Build history of the part. All positions in model axes, mm. A direction names the side the tool comes from. Give positions to 0.01 mm unless a question says otherwise; leave off trailing zeros. Write each loop counter-clockwise with the first axis right and the second up, starting at its lowest first coordinate (ties: lowest second). Pieces come first, ordered by that corner, then holes. Notation, with made-up numbers: (27.25, 57.25) -> (82.25, 57.25) arc R23 cw to (82.25, 88.25) -> close; hole circle Ø4 at (41.5, -14). An arc over 180 degrees is marked (long way). Write item = value, one per line. Start each with the question number.
Q1. Tool access for faces 4 (the face through (-41.214, 41.905, 1.729)), 5 (the face through (135, -24, 11)), 6 (the face through (43.25, 42, 0)), 7 (the face through (155, -10, -10)): list every direction of +Z, -Z, +X, -X, +Y, -Y with a clear straight run to the whole face (end or side of a thin tool).
Q2. Saw through at B-B, the plane y = 21. List the corners of the cut face in (x, z).
Q3. Mould opens along X. For faces 1 (the face through (125.17, -29.38, 0.28)), 2 (the face through (37, 85, -6)), 3 (the face through (135, -24, -11)) say: pulls with the +X half, pulls with the -X half, needs draft (parallel to the pull), parting line crosses it, or undercut.
Q4. Saw through at D-D, the plane y = 53. List the corners of the cut face in (x, z).
Q5. Drop flat-ended pins along their axis: P1, Ø8, axis at x = 31.5, z = 3.5, coming from the -Y side; P2, Ø8, axis at x = 81, z = -21, coming from the +Y side; P3, Ø6.5, axis at x = 40.5, y = 33, coming from the +Z side; P4, Ø8, axis at y = 53, z = 12, coming from the -X side. Give the stop position or say it passes through.
Q6. Saw through at A-A, the plane z = 0. List the corners of the cut face in (x, y), then the cut area to 3 significant figures.
Q7. Wall check: line 1 (Z direction, x = 165, y = 3); line 2 (X direction, y = -20, z = 3); line 3 (X direction, y = -22, z = 10.5). Give the ranges that are in metal, low to high.
Q8. Saw through at C-C, the plane x = 0. List the corners of the cut face in (y, z).
from build123d import *

# Parameters (mm, degrees)
BOSS_EXTRUDE1_DEPTH     = 85
BOSS_EXTRUDE2_START     = -30
SKETCH2_3_R             = 12.5
BOSS_EXTRUDE2_DEPTH     = 56.666666667
EXTRUDE_THIN1_DEPTH     = 115
SKETCH5_W               = 50
SKETCH5_H               = 20
BOSS_EXTRUDE3_DEPTH     = 230
CUT_EXTRUDE2_DEPTH      = 311.201547385
CUT_EXTRUDE2_DEPTH_BACK = 311.201547385
SKETCH5_3_R             = 5
CUT_EXTRUDE1_START      = -30
CUT_EXTRUDE1_OUTLINE_R  = 8.5
CUT_EXTRUDE1_DEPTH      = 115
RIB1_START              = -2.5
RIB1_DEPTH              = 5
FILLET1_R               = 10


# Read off the part's stored shape, not the designer's step: Cut-Extrude1, Rib1
with BuildPart() as part:
    # Sketch2 → Boss-Extrude1 (new body)
    with BuildSketch(Plane(origin=(0, 0, 0), x_dir=(1, 0, 0), z_dir=(0, 1, 0))):
        with BuildLine():
            Line((40.811303581, 6), (46.25, 6))
            Line((46.25, 6), (46.25, -6))
            Line((46.25, -6), (40.811303581, -6))
            ThreePointArc((40.811303581, -6), (-41.25, 0), (40.811303581, 6))
        make_face()
    extrude(amount=BOSS_EXTRUDE1_DEPTH)



with BuildPart() as body_2:
    # Sketch2<3> → Boss-Extrude2 (new body)
    with BuildSketch(Plane(origin=(0, 0, 0), x_dir=(1, 0, 0), z_dir=(0, 1, 0)).offset(BOSS_EXTRUDE2_START)):
        with Locations(Location((165, 0, 0), (0, 0, 270))):
            Circle(SKETCH2_3_R)
    extrude(amount=BOSS_EXTRUDE2_DEPTH)


with BuildPart() as part_1:
    add(part.part)

    add(body_2.part)  # Extrude-Thin1 merges body 2
    # Sketch3 → Extrude-Thin1 (add, symmetric)
    with BuildSketch(Plane.XY):
        Polygon((-41.25, 0), (89.247392222, 0), (125, -30), (177.5, -30), (177.5, -24), (127.183821406, -24), (91.431213628, 6), (-41.25, 6), align=None)
    extrude(amount=EXTRUDE_THIN1_DEPTH, both=True)

    # Sketch5 → Boss-Extrude3 (add)
    with BuildSketch(Plane.XY.offset(115)):
        with Locations((165, -20)):
            Rectangle(SKETCH5_W, SKETCH5_H)
    extrude(amount=-BOSS_EXTRUDE3_DEPTH)

    # Sketch5<3> → Cut-Extrude2 (cut, two sides: drawn at the far end of the back side and taken through both)
    with BuildSketch(Plane.XY.offset(115).offset(-CUT_EXTRUDE2_DEPTH_BACK)):
        with Locations((150, -20)):
            Circle(SKETCH5_3_R)
    extrude(amount=CUT_EXTRUDE2_DEPTH + CUT_EXTRUDE2_DEPTH_BACK, mode=Mode.SUBTRACT)

    # Cut-Extrude1 outline → Cut-Extrude1 (cut)
    with BuildSketch(Plane(origin=(0, 0, 0), x_dir=(1, 0, 0), z_dir=(0, 1, 0)).offset(CUT_EXTRUDE1_START)):
        with BuildLine():
            ThreePointArc((167.178030303, 12.30878483), (174.5779794, 8.03195559), (177.5, 0))
            ThreePointArc((177.5, 0), (174.5779794, -8.03195559), (167.178030303, -12.30878483))
            Line((167.178030303, -12.30878483), (140, -17.117917039))
            Line((140, -17.117917039), (140, -115))
            Line((140, -115), (190, -115))
            Line((190, -115), (190, 115))
            Line((190, 115), (140, 115))
            Line((140, 115), (140, 17.117917039))
            Line((140, 17.117917039), (167.178030303, 12.30878483))
        make_face()
        with BuildLine():
            Line((7.1875, 40.61898994), (140, 17.117917039))
            Line((140, 17.117917039), (140, 115))
            Line((140, 115), (-41.25, 115))
            Line((-41.25, 115), (-41.25, -8.8e-08))
            ThreePointArc((-41.25, -8.8e-08), (-26.505453482, 31.607331993), (7.1875, 40.61898994))
        make_face()
        with BuildLine():
            Line((140, -115), (140, -17.117917039))
            Line((140, -17.117917039), (7.1875, -40.61898994))
            ThreePointArc((7.1875, -40.61898994), (-26.505453415, -31.607332049), (-41.25, -8.8e-08))
            Line((-41.25, -8.8e-08), (-41.25, -115))
            Line((-41.25, -115), (140, -115))
        make_face()
        with Locations((165, 0)):
            Circle(CUT_EXTRUDE1_OUTLINE_R)
        with BuildLine():
            Line((43.25, 3), (37.128998101, 3))
            ThreePointArc((37.128998101, 3), (-37.25, 0), (37.128998101, -3))
            Line((37.128998101, -3), (43.25, -3))
            Line((43.25, -3), (43.25, 3))
        make_face()
    extrude(amount=CUT_EXTRUDE1_DEPTH, mode=Mode.SUBTRACT)

    # Rib1 outline → Rib1 (add)
    with BuildSketch(Plane.XY.offset(RIB1_START)):
        Polygon((145.624979942, 26.666666667), (76.106020374, 85), (46.25, 85), (46.25, 6), (91.431213628, 6), (127.183821406, -24), (140, -24), (140, -10), (154, -10), (154, 26.666666667), align=None)
    extrude(amount=RIB1_DEPTH)

    # Fillet1
    fillet1_edges = [part_1.edges().sort_by_distance(p)[0] for p in [
        (140, -10, 9.80895852),
        (127.183821406, -24, -10.942865145),
        (91.431213628, 6, -14.106063797),
        (145.624979942, 26.666666667, 0),
        (76.106020374, 85, 0),
        (140, -10, -9.808958519),
        (89.247392222, 0, 0),
        (91.431213628, 6, 14.106063797),
        (127.183821406, -24, 10.942865145),
        (125, -30, 0),
    ]]
    fillet(fillet1_edges, radius=FILLET1_R)


solid = part_1.part
Report:
q1.face_4 = +Y
q1.face_5 = +Z, +Y
q1.face_6 = +Y, -Y
q1.face_7 = -Z, +Y
q2.outline = (40.81, -6) -> (46.25, -6) -> (46.25, -2.5) -> (152.75, -2.5) arc R12.5 ccw (long way) to (152.75, 2.5) -> (46.25, 2.5) -> (46.25, 6) -> (40.81, 6) arc R41.25 ccw (long way) to start; hole (37.13, -3) -> (43.25, -3) -> (43.25, 3) -> (37.13, 3) arc R37.25 ccw (long way) to start; hole circle Ø17 at (165, 0)
q3.face_1 = pulls with the -X half
q3.face_2 = needs draft
q3.face_3 = undercut
q4.outline = (40.81, -6) -> (46.25, -6) -> (46.25, -2.5) -> (114.24, -2.5) -> (114.24, 2.5) -> (46.25, 2.5) -> (46.25, 6) -> (40.81, 6) arc R41.25 ccw (long way) to start; hole (37.13, -3) -> (43.25, -3) -> (43.25, 3) -> (37.13, 3) arc R37.25 ccw (long way) to start
q5.P1 = through
q5.P2 = 6
q5.P3 = 17.72
q5.P4 = -40.47
q6.outline = (-41.25, 0) -> (-37.25, 0) -> (-37.25, 85) -> (-41.25, 85) -> close; (43.25, 0) -> (85.61, 0) arc R10 cw to (92.04, -2.34) -> (122.21, -27.66) arc R10 ccw to (128.64, -30) -> (156.5, -30) -> (156.5, 26.67) -> (149.26, 26.67) arc R10 cw to (142.84, 29.01) -> (78.89, 82.66) arc R10 ccw to (72.47, 85) -> (43.25, 85) -> close; (173.5, -30) -> (177.5, -30) -> (177.5, 26.67) -> (173.5, 26.67) -> close; hole circle Ø10 at (150, -20)
q6.area = 8,930 mm2
q7.line_1 = -12.5 to -8.5, 8.5 to 12.5
q7.line_2 = 113.08 to 122.42, 140 to 145, 155 to 157.05, 172.95 to 177.13
q7.line_3 = 115.47 to 124.82, 140 to 145.42, 154.58 to 171.78
q8.outline = (0, -41.25) -> (85, -41.25) -> (85, -37.25) -> (0, -37.25) -> close; (0, 37.25) -> (85, 37.25) -> (85, 41.25) -> (0, 41.25) -> close
